Print and shaded views of the part. All mm, measured from the part's lowest x, y and z. Round coordinates to 2 decimals unless told otherwise and drop trailing zeros. Loops run counter-clockwise (first coordinate to the right, second up) from the corner with the lowest first, then second, coordinate; pieces in that order, holes last. Notation, with made-up numbers: (43, -37.75) - (56, -37.75) arc R26 cw to (56, -20.75) - close; hole circle Ø7 at (-21.75, -31). An arc over 180 degrees is marked (long way). Use one line per item in the form item = value.
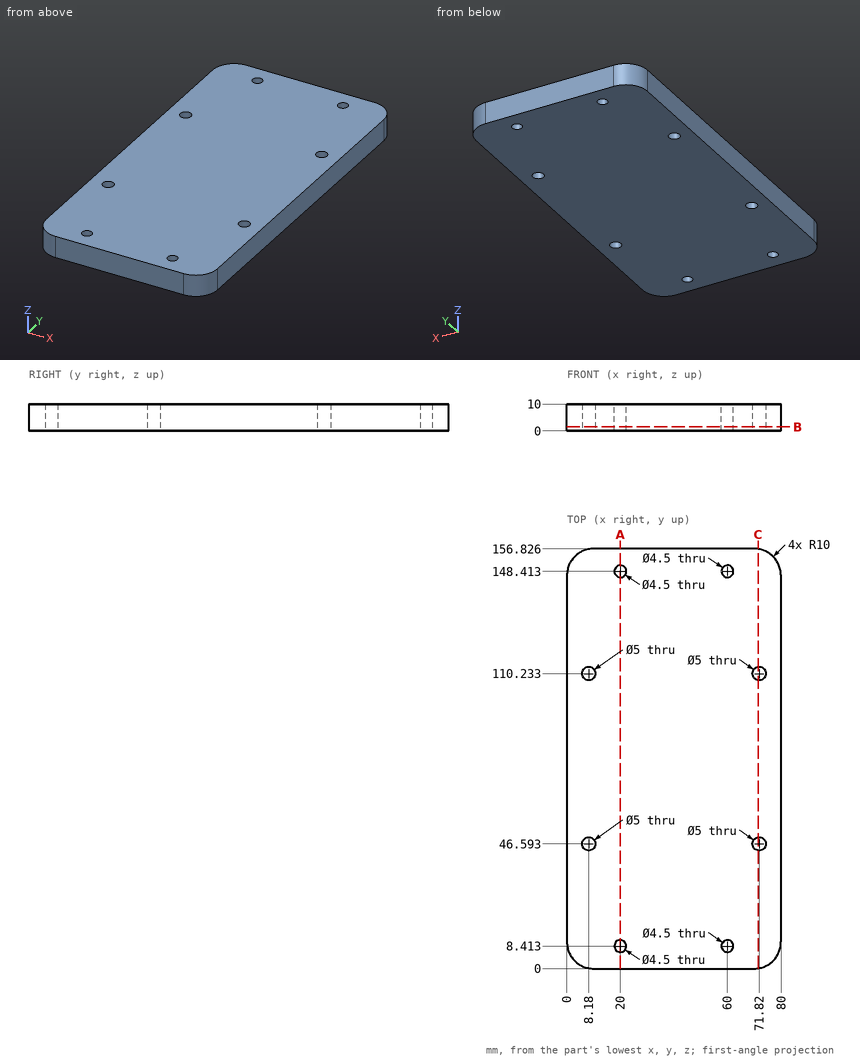
1. Cut at B-B, the plane z = 1.5. Give the number of separate pieces and of enclosed holes in the cut face, plus the area to 3 significant figures.
Geometry check:
separate_pieces = 1
enclosed_holes = 8
area = 12,300 mm^2
2. Flat gauge pin, fed straight in: pin 1 (4.5 mm diameter, centred on x = 71.82, y = 46.59, fed in from -Z). Where does the tip first touch, or does it go through?
Geometry check:
pin_1 = through
3. Wall check: probe 1 along X at (y, z) = (46.5, 3.5); probe 2 along Y at (x, z) = (60, 8) (1 decimal); probe 3 along X at (y, z) = (146.5, 0.5) (1 decimal). Give the ranges that are in metal, low to high.
Geometry check:
probe_1 = 0 to 5.68, 10.68 to 69.32, 74.32 to 80
probe_2 = 0 to 6.2, 10.7 to 146.2, 150.7 to 156.8
probe_3 = 0 to 18.8, 21.2 to 58.8, 61.2 to 80
4. Cut at C-C, the plane x = 71.5. Give the cut face in (y, z), plus the area to 3 significant figures.
Geometry check:
outline = (0.11, 0) - (44.11, 0) - (44.11, 10) - (0.11, 10) - close; (49.07, 0) - (107.75, 0) - (107.75, 10) - (49.07, 10) - close; (112.71, 0) - (156.71, 0) - (156.71, 10) - (112.71, 10) - close
area = 1,470 mm^2
5. Cut at A-A, the plane x = 20. Give the cut face in (y, z) (1 decimal).
Geometry check:
outline = (0, 0) - (6.2, 0) - (6.2, 10) - (0, 10) - close; (10.7, 0) - (146.2, 0) - (146.2, 10) - (10.7, 10) - close; (150.7, 0) - (156.8, 0) - (156.8, 10) - (150.7, 10) - close
